```python
from build123d import *

# Parameters (mm, degrees)
SKETCH1_R           = 12
BOSS_EXTRUDE1_DEPTH = 2
SKETCH2_R           = 12.5
SKETCH2_R_2         = 11.5
BOSS_EXTRUDE2_DEPTH = 0.7
SKETCH3_R           = 3
CUT_EXTRUDE1_DEPTH  = 18.790446875
SKETCH4_R           = 7.5
BOSS_EXTRUDE4_DEPTH = 2.7
SKETCH5_R           = 3
CUT_EXTRUDE3_DEPTH  = 19.291801442


with BuildPart() as part:
    # Sketch1 → Boss-Extrude1 (new body)
    with BuildSketch(Plane.XY):
        Circle(SKETCH1_R)
    extrude(amount=BOSS_EXTRUDE1_DEPTH)

    # Sketch2 → Boss-Extrude2 (add)
    with BuildSketch(Plane(origin=(0, 0, 0), x_dir=(-1, 0, 0), z_dir=(0, 0, -1))):
        Circle(SKETCH2_R)
        Circle(SKETCH2_R_2, mode=Mode.SUBTRACT)
    extrude(amount=BOSS_EXTRUDE2_DEPTH)

    # Sketch3 → Cut-Extrude1 (cut, through all)
    with BuildSketch(Plane(origin=(0, 0, 0), x_dir=(-1, 0, 0), z_dir=(0, 0, -1))):
        Circle(SKETCH3_R)
    extrude(amount=-CUT_EXTRUDE1_DEPTH, mode=Mode.SUBTRACT)

    # Sketch4 → Boss-Extrude4 (add)
    with BuildSketch(Plane(origin=(0, 0, 0), x_dir=(-1, 0, 0), z_dir=(0, 0, -1))):
        with Locations(Location((0, 0, 0), (0, 0, 180))):
            Circle(SKETCH4_R)
    extrude(amount=BOSS_EXTRUDE4_DEPTH)

    # Sketch5 → Cut-Extrude3 (cut, through all)
    with BuildSketch(Plane(origin=(0, 0, -2.7), x_dir=(-1, 0, 0), z_dir=(0, 0, -1))):
        Circle(SKETCH5_R)
    extrude(amount=-CUT_EXTRUDE3_DEPTH, mode=Mode.SUBTRACT)


solid = part.part
```
Can you work these out from the model? Positions are in its coordinate system, mm. A direction names the side the tool comes from. Round coordinates to 2 decimals unless told otherwise and drop trailing zeros. Order: outer loops, then holes, each group sorted by start corner. A loop starts at its lowest first (then second) coordinate and runs counter-clockwise, first axis right, second up. Notation, with made-up numbers: (73, 47) -> (89, 47) arc R29 cw to (89, 69) -> close; hole circle Ø7 at (70.5, 35). An arc over 180 degrees is marked (long way). Return JSON: item names as keys, results as strings. Group by question number.
1. If we section it at A-A, the plane y = 0: Write out the boundary of the cut face in (x, z), then the cut area to 3 significant figures.
2. If we section it at C-C, the plane z = -2.4: Write out the boundary of the cut face in (x, y), then the cut area to 3 significant figures.
3. I need wall thicknesses on line 1 (Y direction, x = 0, z = -0.1); line 2 (Y direction, x = 0, z = 0.8); line 3 (Y direction, x = 0, z = -1.4). Which ranges of each line are inside material? Lowest first, please. Write a range as [from, to].
4. We'd pull the mould along Y, two halves only. Please class faces 4 (the face through (-11.923, 3.755, -0.345)), 5 (the face through (3, 0, 0)), 6 (the face through (-11, -4, -0.7)): released by +Y, released by -Y, zero draft, split by the parting line, or undercut.
5. Will this pin go through, and if not, where does the flat tip stop? pin 1 (1.5 mm diameter, centred on y = -3, z = 1, fed in from -X).
6. Which directions (+Z, -Z, +X, -X, +Y, -Y) give clear straight access to the entire face, cutting with the end or side of a thin tool? Please do faces 1 (the face through (0, -8, 0)), 2 (the face through (3.2, -0.1, -2.7)), 3 (the face through (7, 10, 0)).
7. If we section it at D-D, the plane x = -3.75: Write out the boundary of the cut face in (y, z).
Output values:
{
 "1": {"outline": "(-12.5, -0.7) -> (-11.5, -0.7) -> (-11.5, 0) -> (-7.5, 0) -> (-7.5, -2.7) -> (-3, -2.7) -> (-3, 2) -> (-12, 2) -> (-12, 0) -> (-12.5, 0) -> close; (3, -2.7) -> (7.5, -2.7) -> (7.5, 0) -> (11.5, 0) -> (11.5, -0.7) -> (12.5, -0.7) -> (12.5, 0) -> (12, 0) -> (12, 2) -> (3, 2) -> close", "area": "61.7 mm²"},
 "2": {"outline": "circle Ø15 at (0, 0); hole circle Ø6 at (0, 0)", "area": "148 mm²"},
 "3": {"line 1": "[-12.5, -11.5], [-7.5, -3], [3, 7.5], [11.5, 12.5]", "line 2": "[-12, -3], [3, 12]", "line 3": "[-7.5, -3], [3, 7.5]"},
 "4": {"face 4": "split by the parting line", "face 5": "undercut", "face 6": "zero draft"},
 "5": {"pin 1": "x = -11.79"},
 "6": {"face 1": "-Z", "face 2": "-Z, +X, -X, +Y, -Y", "face 3": "+Z"},
 "7": {"outline": "(-11.92, -0.7) -> (-10.87, -0.7) -> (-10.87, 0) -> (-6.5, 0) -> (-6.5, -2.7) -> (6.5, -2.7) -> (6.5, 0) -> (10.87, 0) -> (10.87, -0.7) -> (11.92, -0.7) -> (11.92, 0) -> (11.4, 0) -> (11.4, 2) -> (-11.4, 2) -> (-11.4, 0) -> (-11.92, 0) -> close"}
}
